Answer from the drawing. Dimensions are ordinates in mm from the lowest x, y and z of the part. Round coordinates to 2 decimals unless told otherwise and drop trailing zeros. Write each loop counter-clockwise with the first axis right and the second up, starting at its lowest first coordinate (ties: lowest second). Pieces come first, ordered by that corner, then holes.
1. Straight lines are drawn through the part: probe 1 along Y at (x, z) = (39.29, 0.75); probe 2 along Y at (x, z) = (10.21, 1.4); probe 3 along Z at (x, y) = (28, 20). For each, find the intervals that lie inside material, in ascending order.
2. Find section A-A (z = 3.5). Write down the section's boundary in (x, y).
3. Flat-ended cylindrical pins translate along their axes: pin 1 Ø16.5 at (x, y) = (17, 8.5) entering from +Z; pin 2 Ø1 at (x, z) = (1, 3) entering from -Y; pin 3 Ø0.6 at (x, z) = (48.5, 4) entering from +Y. Find the tip coordinate at first contact, or state that the pin passes through.
4. Find section D-D (x = 39.29). Write down the section's boundary in (y, z).
5. Find section B-B (x = 10.21). Write down the section's boundary in (y, z).
6. Find section C-C (y = 16.5). Write down the section's boundary in (x, z).
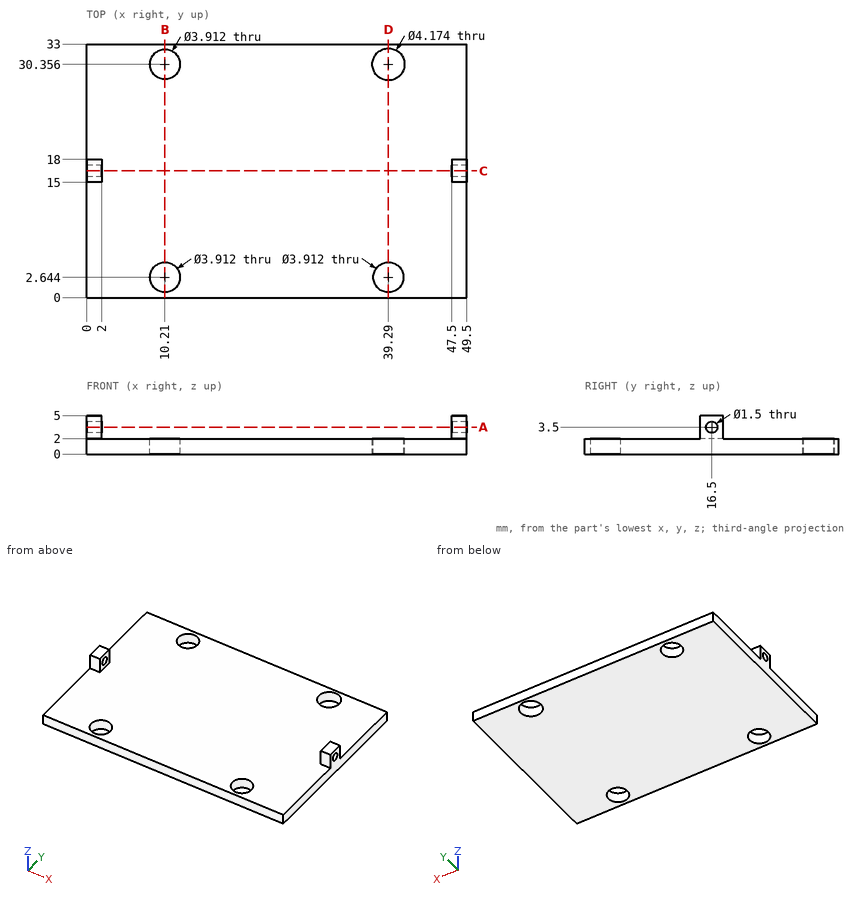
Worked answers:
1. probe 1: y = 0 to 0.69, 4.6 to 28.27, 32.44 to 33
1. probe 2: y = 0 to 0.69, 4.6 to 28.4, 32.31 to 33
1. probe 3: z = 0 to 2
2. outline: (0, 15) - (2, 15) - (2, 15.75) - (0, 15.75) - close; (0, 17.25) - (2, 17.25) - (2, 18) - (0, 18) - close; (47.5, 15) - (49.5, 15) - (49.5, 15.75) - (47.5, 15.75) - close; (47.5, 17.25) - (49.5, 17.25) - (49.5, 18) - (47.5, 18) - close
3. pin 1: stops at z = 2
3. pin 2: stops at y = 15
3. pin 3: stops at y = 18
4. outline: (0, 0) - (0.69, 0) - (0.69, 2) - (0, 2) - close; (4.6, 0) - (28.27, 0) - (28.27, 2) - (4.6, 2) - close; (32.44, 0) - (33, 0) - (33, 2) - (32.44, 2) - close
5. outline: (0, 0) - (0.69, 0) - (0.69, 2) - (0, 2) - close; (4.6, 0) - (28.4, 0) - (28.4, 2) - (4.6, 2) - close; (32.31, 0) - (33, 0) - (33, 2) - (32.31, 2) - close
6. outline: (0, 0) - (49.5, 0) - (49.5, 2.75) - (47.5, 2.75) - (47.5, 2) - (2, 2) - (2, 2.75) - (0, 2.75) - close; (0, 4.25) - (2, 4.25) - (2, 5) - (0, 5) - close; (47.5, 4.25) - (49.5, 4.25) - (49.5, 5) - (47.5, 5) - close
